Design review of the part built by this model. Coordinates are the model's own, in mm. A direction names the side the tool comes from. Coordinates: 2 decimals unless noted, no trailing zeros. Loops run counter-clockwise (first coordinate to the right, second up) from the corner with the lowest first, then second, coordinate; pieces in that order, holes last. Notation, with made-up numbers: M -36.75,66.5 L 8.25,66.5 A9 cw 8.25,78.5 Z; hole C 47.5,5 d2. An arc over 180 degrees is marked long. One line per item, written item: value.
```python
from build123d import *

# Parameters (mm, degrees)
F0_R     = 37.5158
F2_DEPTH = 63.5
F1_R     = 39.7256
F3_DEPTH = 63.5
F4_R     = 2.5654
F4_R_2   = 2.6035
F4_R_3   = 3.5941
F4_R_4   = 3.2766
F4_R_5   = 4.7879
F5_DEPTH = 127.001
F6_R     = 31.165799
F6_R_2   = 4.7879
F6_R_3   = 3.2766
F6_R_4   = 3.5941
F6_R_5   = 2.6035
F6_R_6   = 2.5654
F7_DEPTH = 101.6


with BuildPart() as f2:
    # F0 (on Front) → F2 (new body)
    with BuildSketch(Plane.XZ):
        Circle(F0_R)
    extrude(amount=F2_DEPTH)

    # F1 (on Front) → F3 (join)
    with BuildSketch(Plane.XZ):
        Circle(F1_R)
    extrude(amount=-F3_DEPTH)

    # F4 (on face) → F5 (cut, through all)
    with BuildSketch(Plane(origin=(0, 63.5, 0), x_dir=(-1, 0, 0), z_dir=(0, 1, 0))):
        with Locations((0, 21.9456)):
            Circle(F4_R)
        with Locations((-19.545753, 9.978621)):
            Circle(F4_R_2)
        with Locations((20.072576, 8.871361)):
            Circle(F4_R_3)
        with Locations((-12.724472, -17.880078)):
            Circle(F4_R_4)
        with Locations((16.162698, -14.845085)):
            Circle(F4_R_5)
    extrude(amount=-F5_DEPTH, mode=Mode.SUBTRACT)

    # F6 (on face) → F7 (cut)
    with BuildSketch(Plane.XZ.offset(63.5)):
        Circle(F6_R)
        with Locations((-16.162698, -14.845085)):
            Circle(F6_R_2, mode=Mode.SUBTRACT)
        with Locations((12.724472, -17.880078)):
            Circle(F6_R_3, mode=Mode.SUBTRACT)
        with Locations((-20.072576, 8.871361)):
            Circle(F6_R_4, mode=Mode.SUBTRACT)
        with Locations((19.545753, 9.978621)):
            Circle(F6_R_5, mode=Mode.SUBTRACT)
        with Locations((0, 21.9456)):
            Circle(F6_R_6, mode=Mode.SUBTRACT)
    extrude(amount=-F7_DEPTH, mode=Mode.SUBTRACT)


solid = f2.part
```
(1) Mouldability with a two-part tool opening along X and no side actions: class faces 1 (the cylindrical face through (35.783, -31.306, 11.269)), 2 (the cylindrical face through (10.96, 50.98, -15.12)), 3 (the cylindrical face through (-12.363, 50.978, -17.758)), 4 (the flat face through (5, -63.5, 31)) as released by +X, released by -X, zero draft, split by the parting line, or undercut.
Reply:
face 1: split by the parting line
face 2: undercut
face 3: undercut
face 4: zero draft
(2) We need section B-B on x = -19. State the section outline as (y, z) points, then the cut area to 3 significant figures.
Reply:
outline: M -63.5,-32.35 L 0,-32.35 L 0,-34.89 L 63.5,-34.89 L 63.5,-18.7 L 38.1,-18.7 L 38.1,-24.7 L -63.5,-24.7 Z; M -63.5,24.7 L 38.1,24.7 L 38.1,12.3 L 63.5,12.3 L 63.5,34.89 L 0,34.89 L 0,32.35 L -63.5,32.35 Z; M 38.1,-10.99 L 63.5,-10.99 L 63.5,5.44 L 38.1,5.44 Z
area: 3,150 mm2
(3) We need section A-A on x = 0. State the section outline as (y, z) points.
Reply:
outline: M -63.5,-37.52 L 0,-37.52 L 0,-39.73 L 63.5,-39.73 L 63.5,19.38 L 38.1,19.38 L 38.1,-31.17 L -63.5,-31.17 Z; M -63.5,31.17 L 38.1,31.17 L 38.1,24.51 L 63.5,24.51 L 63.5,39.73 L 0,39.73 L 0,37.52 L -63.5,37.52 Z
(4) Insertion check: pin 1 (2 mm diameter, centred on x = 30.5, y = -18, fed in from +Z); pin 2 (6 mm diameter, centred on x = 18.5, y = 44.5, fed in from -Z); pin 3 (6 mm diameter, centred on y = -13, z = -20, fed in from -X); pin 4 (4 mm diameter, centred on x = 19.55, z = 9.98, fed in from -Y). Each pin has a flat end and moves straight along its axis. Give the tip position at first contact, or say it passes through.
Reply:
pin 1: stops at z = 23.18
pin 2: stops at z = -36.58
pin 3: stops at x = -33.44
pin 4: passes through
(5) Tool access review of faces 5 (the flat face through (15, 0, -35)), 6 (the flat face through (-1, 63.5, 1)): name each direction out of +Z, -Z, +X, -X, +Y, -Y from which nothing blocks a thin tool from reaching the whole face with its end or side.
Reply:
face 5: -Y
face 6: +Z, -Z, +X, -X, +Y
(6) We need section C-C on z = 0. State the section outline as (x, y) points, then the cut area to 3 significant figures.
Reply:
outline: M -39.73,0 L -37.52,0 L -37.52,-63.5 L -31.17,-63.5 L -31.17,38.1 L 31.17,38.1 L 31.17,-63.5 L 37.52,-63.5 L 37.52,0 L 39.73,0 L 39.73,63.5 L -39.73,63.5 Z
area: 3,480 mm2
(7) To check wall thickness, follow line 1 along Z through (x, y) = (0, -30); line 2 along Y through (x, z) = (-30.5, -6); line 3 along X through (y, z) = (-37, -20.5). State the ranges of each line that lie inside material, in increasing order. Write a range as [from, to].
Reply:
line 1: z = [-37.52, -31.17], [31.17, 37.52]
line 2: y = [38.1, 63.5]
line 3: x = [-31.42, -23.47], [23.47, 31.42]
(8) We need section D-D on y = 33. State the section outline as (x, z) points, then the cut area to 3 significant figures.
Reply:
outline: C 0,0 d79.45; hole C 0,0 d62.33
area: 1,910 mm2
